Geometry check sheet. Reference: the model listing, model coordinates, mm. A direction names the side the tool comes from. Round coordinates to 2 decimals unless told otherwise and drop trailing zeros. Write each loop counter-clockwise with the first axis right and the second up, starting at its lowest first coordinate (ties: lowest second). Pieces come first, ordered by that corner, then holes. Notation, with made-up numbers: (64.25, -30) - (102.25, -30) arc R15 cw to (102.25, -11) - close; hole circle Ø9 at (-6, 80.5). An arc over 180 degrees is marked (long way). Return JSON: item names as keys, results as strings.
Autodesk Inventor part; units mm, degrees
ref_plane "YZ Plane" through (0, 0, 0) normal (1, 0, 0) x (0, 1, 0)
ref_plane "XZ Plane" through (0, 0, 0) normal (0, 1, 0) x (-1, 0, 0)
ref_plane "XY Plane" through (0, 0, 0) normal (0, 0, 1) x (1, 0, 0)
sketch "Sketch1" plane through (0, 0, 0) normal (0, 0, 1) x (1, 0, 0)
  circle A0 centre (0, 0) radius 15.875
  line L0 (0, 0) -> (-127, 0)
  circle A1 centre (-127, 0) radius 15.875
  line L1 (-127, 15.875) -> (0, 15.875)
  line L2 (0, -15.875) -> (-127, -15.875)
  circle A2 centre (-127, 0) radius 2.1082
  dimension "d0" = 31.75
  dimension "d1" = 127
  dimension "d2" = 31.75
  dimension "d3" = 4.2164
extrude "Extrusion1" add sketch "Sketch1" along normal blind 3.175
sketch "Sketch2" plane through (0, 0, 0) normal (0, 0, -1) x (-1, 0, 0)
  arc A0 (127, -15.875) -> (127, 15.875) centre (127, 0) ccw
  line L0 (0, 15.875) -> (127, 15.875)
  arc A1 (0, 15.875) -> (0, -15.875) centre (0, 0) ccw
  line L1 (127, -15.875) -> (0, -15.875)
  circle A2 centre (127, 0) radius 2.1082
  line L2 (121.959, 0) -> (124.4795, 4.3656)
  line L3 (124.4795, 4.3656) -> (129.5205, 4.3656)
  line L4 (129.5205, 4.3656) -> (132.041, 0)
  line L5 (132.041, 0) -> (129.5205, -4.3656)
  line L6 (129.5205, -4.3656) -> (124.4795, -4.3656)
  line L7 (124.4795, -4.3656) -> (121.959, 0)
  dimension "d6" = 4.3656
extrude "Extrusion2" add sketch "Sketch2" along normal blind 3.175 contours L1 A1 L0 A0
fillet "Fillet1" radius 3.175 4 edges at (15.875, 0, -3.175) (-63.5, -15.875, -3.175) (-142.875, 0, -3.175) (-63.5, 15.875, -3.175)
sketch "Sketch3" plane through (0, 0, 3.175) normal (0, 0, 1) x (1, 0, 0)
  arc A0 (-127, 15.875) -> (-127, -15.875) centre (-127, 0) ccw
  line L0 (-127, -15.875) -> (0, -15.875)
  arc A1 (0, -15.875) -> (0, 15.875) centre (0, 0) ccw
  line L1 (0, 15.875) -> (-127, 15.875)
  circle A2 centre (-127, 0) radius 2.1082
  circle A3 centre (-127, 0) radius 3.9688
  dimension "d10" = 7.9375
extrude "Extrusion3" add sketch "Sketch3" along normal blind 3.175 contours L1 A1 L0 A0
sketch "Sketch4" plane through (0, 0, 6.35) normal (0, 0, 1) x (1, 0, 0)
  line L0 (-127, -15.875) -> (0, -15.875)
  arc A0 (0, -15.875) -> (0, 15.875) centre (0, 0) ccw
  line L1 (0, 15.875) -> (-127, 15.875)
  arc A1 (-127, 15.875) -> (-127, -15.875) centre (-127, 0) ccw
  circle A2 centre (-127, 0) radius 3.9688
  circle A3 centre (-127, 0) radius 2.1082
  circle A4 centre (-127, 0) radius 11.1125
  circle A5 centre (0, 0) radius 11.1125
  dimension "d13" = 22.225
  dimension "d14" = 22.225
extrude "Extrusion4" add sketch "Sketch4" along normal blind 5.5372 contours A1 L1 A0 L0
sketch "Sketch5" plane through (0, 0, 11.8872) normal (0, 0, 1) x (1, 0, 0)
  circle A0 centre (-76.2, 0) radius 2.1082
  circle A1 centre (-50.8, 0) radius 2.1082
  circle A2 centre (-127, 0) radius 2.1082
  point P0 (0, 0)
  dimension "d17" = 4.2164
  dimension "d18" = 4.2164
  dimension "d19" = 50.8
  dimension "d20" = 50.8
extrude "Extrusion5" cut sketch "Sketch5" against normal blind 25.4 contours A0 | A1
fillet "Fillet2" radius 1.5875 4 edges at (-142.875, 0, 11.8872) (-63.5, -15.875, 11.8872) (15.875, 0, 11.8872) (-63.5, 15.875, 11.8872)
fillet "Fillet3" radius 1.5875 1 edges at (-130.9688, 0, 6.35)
properties part number "Plate E"
(1) Access from +Z, -Z, +X, -X, +Y, -Y to the whole of each face (thin tool, end or side, straight path). Record for faces 4 (the face through (-132, 3, 6.35)), 5 (the face through (-127, 4.366, -2)), 6 (the face through (-65, 0, 11.887)).
Response values:
{"face 4": "+Z", "face 5": "-Z", "face 6": "+Z, +X, -X, +Y, -Y"}
(2) Material ranges on line 1 along Y through (x, z) = (-50.8, 6) (3 decimals); line 2 along X through (y, z) = (-6, 10.75); line 3 along Z through (x, y) = (-123, 3.5) (3 decimals), recorded low to high. Write a range as [from, to].
Response values:
{"line 1": "y = [-15.875, -2.108], [2.108, 15.875]", "line 2": "x = [-141.63, -136.35], [-117.65, -9.35], [9.35, 14.63]", "line 3": "z = [-3.175, 6.332]"}
(3) Gauge pin test, flat ends, axial feed: pin 1 (1 mm diameter, centred on x = -127.5, z = -1, fed in from +Y); pin 2 (8.5 mm diameter, centred on x = -129, y = -1.5, fed in from +Z); pin 3 (9.5 mm diameter, centred on x = -125.5, y = 0.5, fed in from -Z) (3 decimals); pin 4 (3 mm diameter, centred on y = -7.5, z = 6, fed in from -X). Record the tip position at first contact, or that the pin passes through.
Response values:
{"pin 1": "stops at y = 15.83", "pin 2": "stops at z = 6.35", "pin 3": "stops at z = -3.175", "pin 4": "stops at x = -141.7"}
(4) Release check for a two-part mould opening along Y. For faces 1 (the face through (-62.61, 14.92, -2.27)), 2 (the face through (-142.87, -0.35, 5.08)), 3 (the face through (-130.763, 2.213, -1.565)) record: pulls with the +Y half, pulls with the -Y half, needs draft (parallel to the pull), parting line crosses it, or undercut.
Response values:
{"face 1": "pulls with the +Y half", "face 2": "parting line crosses it", "face 3": "undercut"}
(5) Section check A-A, the plane x = -76.2. Enter the section's corners in (y, z) (1 decimal).
Response values:
{"outline": "(-15.9, 0) arc R3.2 ccw to (-12.7, -3.2) - (-2.1, -3.2) - (-2.1, 11.9) - (-14.3, 11.9) arc R1.6 ccw to (-15.9, 10.3) - close; (2.1, -3.2) - (12.7, -3.2) arc R3.2 ccw to (15.9, 0) - (15.9, 10.3) arc R1.6 ccw to (14.3, 11.9) - (2.1, 11.9) - close"}
(6) Section check B-B, the plane z = -1.5. Enter the section's corners in (x, y), plus the area to 3 significant figures.
Response values:
{"outline": "(-127, -15.5) - (0, -15.5) arc R15.5 ccw to (0, 15.5) - (-127, 15.5) arc R15.5 ccw to start; hole (-132.04, 0) - (-129.52, -4.37) - (-124.48, -4.37) - (-121.96, 0) - (-124.48, 4.37) - (-129.52, 4.37) - close; hole circle Ø4.22 at (-76.2, 0); hole circle Ø4.22 at (-50.8, 0)", "area": "4,600 mm^2"}
